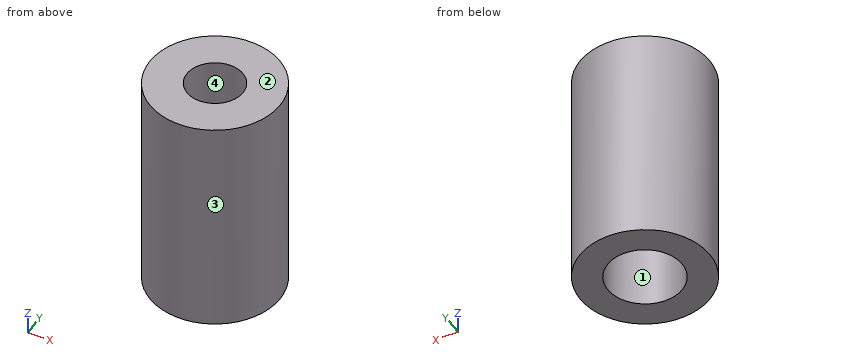
```python
from build123d import *

# Parameters (mm, degrees)
ESQUISSE1_R             = 17.5
BOSS_EXTRU_1_DEPTH      = 30
ENL_V_START             = -30
ESQUISSE2_R             = 7.55
ENL_V_MAT_EXTRU_1_DEPTH = 30
ESQUISSE3_R             = 10.05
ENL_V_MAT_EXTRU_2_DEPTH = 30


with BuildPart() as part:
    # Esquisse1 → Boss.-Extru.1 (new body, symmetric)
    with BuildSketch(Plane.XY):
        Circle(ESQUISSE1_R)
    extrude(amount=BOSS_EXTRU_1_DEPTH, both=True)

    # Esquisse2 → Enlèv. mat.-Extru.1 (cut)
    with BuildSketch(Plane.XY.offset(30).offset(ENL_V_START)):
        Circle(ESQUISSE2_R)
    extrude(amount=ENL_V_MAT_EXTRU_1_DEPTH, mode=Mode.SUBTRACT)

    # Esquisse3 → Enlèv. mat.-Extru.2 (cut)
    with BuildSketch(Plane(origin=(0, 0, -30), x_dir=(-1, 0, 0), z_dir=(0, 0, -1)).offset(ENL_V_START)):
        Circle(ESQUISSE3_R)
    extrude(amount=ENL_V_MAT_EXTRU_2_DEPTH, mode=Mode.SUBTRACT)


solid = part.part
```
Check sheet for the modelled part. Datum: model origin and axes. Units: mm. Face numbers are marked on the shaded views. Coordinates: 2 decimals unless noted, no trailing zeros. Order: outer loops, then holes, each group sorted by start corner. A loop starts at its lowest first (then second) coordinate and runs counter-clockwise, first axis right, second up. Notation, with made-up numbers: M 4.5,47.5 L 35.5,47.5 A22 ccw 35.5,68.5 Z; hole C 77.5,65.25 d9. An arc over 180 degrees is marked long. One line per question, with ' | ' between items. Start each with the question number.
Item 1: Sectioned sample at C-C on z = 14. Record the cut outline in (x, y), and give its area (3 significant figures).
Item 2: Material ranges on line 1 (Y direction, x = 0, z = -9.5); line 2 (Y direction, x = 0, z = 16); line 3 (Z direction, x = 2, y = -7.5), recorded low to high.
Item 3: Sectioned sample at D-D on y = -9. Record the cut outline in (x, z).
Item 4: Sectioned sample at A-A on x = 0. Record the cut outline in (y, z), and give its area (3 significant figures).
Item 5: Mould release check, pull along X, two halves, no side actions. Record for the marked faces 1, 2, 3 and 4: pulls with the +X half, pulls with the -X half, needs draft (parallel to the pull), parting line crosses it, or undercut.
Item 6: Gauge pin test, flat ends, axial feed: P1, Ø10, axis at x = 0.5, y = -4, coming from the -Z side; P2, Ø1.5, axis at y = 12.5, z = -7.5, coming from the -X side; P3, Ø1, axis at y = 9, z = 14, coming from the +X side. Record the tip position at first contact, or that the pin passes through.
Answer below:
1) outline: C 0,0 d35; hole C 0,0 d15.1 | area: 783 mm^2
2) line 1: y = -17.5 to -10.05, 10.05 to 17.5 | line 2: y = -17.5 to -7.55, 7.55 to 17.5 | line 3: z = 0 to 30
3) outline: M -15.01,-30 L -4.47,-30 L -4.47,0 L 4.47,0 L 4.47,-30 L 15.01,-30 L 15.01,30 L -15.01,30 Z
4) outline: M -17.5,-30 L -10.05,-30 L -10.05,0 L -7.55,0 L -7.55,30 L -17.5,30 Z; M 7.55,0 L 10.05,0 L 10.05,-30 L 17.5,-30 L 17.5,30 L 7.55,30 Z | area: 1,040 mm^2
5) face 1: undercut | face 2: needs draft | face 3: parting line crosses it | face 4: undercut
6) P1: stops at z = 0 | P2: stops at x = -12.97 | P3: stops at x = 15.3
